Source: CAD feature listing. Evaluate the final solid. Frame: model axes, mm. A direction names the side the tool comes from. Give positions to 0.01 mm unless a question says otherwise; leave off trailing zeros. Loops run counter-clockwise (first coordinate to the right, second up) from the corner with the lowest first, then second, coordinate; pieces in that order, holes last. Notation, with made-up numbers: M -35.5,-14 L -20.5,-14 A27 ccw -20.5,16 Z; hole C -8,-7 d5. An arc over 180 degrees is marked long. Answer in a Markdown table with one row per item.
Autodesk Inventor part; units mm, degrees
ref_plane "YZ Plane" through (0, 0, 0) normal (1, 0, 0) x (0, 1, 0)
ref_plane "XZ Plane" through (0, 0, 0) normal (0, 1, 0) x (-1, 0, 0)
ref_plane "XY Plane" through (0, 0, 0) normal (0, 0, 1) x (1, 0, 0)
sketch "Sketch1" plane through (0, 0, 0) normal (0, 0, 1) x (1, 0, 0)
  line L0 (87.39809, 90.638849) -> (76.791489, 101.245451)
  line L1 (110.603697, 90.638591) -> (87.39809, 90.638849)
  line L2 (121.210063, 101.244956) -> (110.603697, 90.638591)
  line L3 (143.419374, 101.244709) -> (121.210063, 101.244956)
  line L4 (153.419263, 111.244598) -> (143.419374, 101.244709)
  line L5 (153.419473, 130.081843) -> (153.419263, 111.244598)
  line L6 (144.001258, 139.500058) -> (153.419473, 130.081843)
  line L7 (144.001258, 184.500058) -> (144.001258, 139.500058)
  line L8 (162.838724, 203.336883) -> (144.001258, 184.500058)
  line L9 (174.479779, 203.336684) -> (162.838724, 203.336883)
  line L10 (188.623093, 217.476415) -> (174.479779, 203.336684)
  line L11 (188.623904, 237.476415) -> (188.623093, 217.476415)
  line L12 (174.481567, 251.622561) -> (188.623904, 237.476415)
  line L13 (154.481567, 251.622902) -> (174.481567, 251.622561)
  line L14 (140.33919, 237.481007) -> (154.481567, 251.622902)
  line L15 (140.338992, 225.83779) -> (140.33919, 237.481007)
  line L16 (121.502223, 207.001664) -> (140.338992, 225.83779)
  line L17 (76.502223, 207.001664) -> (121.502223, 207.001664)
  line L18 (57.665842, 225.839164) -> (76.502223, 207.001664)
  line L19 (57.66604, 237.480627) -> (57.665842, 225.839164)
  line L20 (43.524145, 251.623004) -> (57.66604, 237.480627)
  line L21 (23.524145, 251.623344) -> (43.524145, 251.623004)
  line L22 (9.381769, 237.48145) -> (23.524145, 251.623344)
  line L23 (9.380958, 217.48145) -> (9.381769, 237.48145)
  line L24 (23.52252, 203.338741) -> (9.380958, 217.48145)
  line L25 (35.165328, 203.338269) -> (23.52252, 203.338741)
  line L26 (54.001421, 184.501058) -> (35.165328, 203.338269)
  line L27 (54.001421, 139.501058) -> (54.001421, 184.501058)
  line L28 (44.582671, 130.082867) -> (54.001421, 139.501058)
  line L29 (44.582461, 111.245809) -> (44.582671, 130.082867)
  line L30 (54.582226, 101.245698) -> (44.582461, 111.245809)
  line L31 (76.791489, 101.245451) -> (54.582226, 101.245698)
  circle A0 centre (99, 132) radius 5.5
  arc A1 (130.06, 142) -> (135.06, 142) centre (132.56, 142) ccw
  line L32 (130.06, 142) -> (130.06, 182)
  line L33 (135.06, 182) -> (135.06, 142)
  arc A2 (62.940969, 142) -> (67.940969, 142) centre (65.440969, 142) ccw
  arc A3 (67.940969, 182) -> (62.940969, 182) centre (65.440969, 182) ccw
  line L34 (67.940969, 182) -> (67.940969, 142)
  line L35 (138.997508, 214.221497) -> (150.997508, 202.221497)
  line L36 (128.721743, 214.221497) -> (138.997508, 214.221497)
  line L37 (121.5, 207) -> (128.721743, 214.221497)
  line L38 (76.5, 207) -> (121.5, 207)
  line L39 (69.278592, 214.221497) -> (76.5, 207)
  line L40 (59.002492, 214.221497) -> (69.278592, 214.221497)
  line L41 (47.002492, 202.221497) -> (59.002492, 214.221497)
  line L42 (47.002492, 191.497594) -> (47.002492, 202.221497)
  line L43 (54, 184.5) -> (47.002492, 191.497594)
  line L44 (54, 139.5) -> (54, 184.5)
  line L45 (47.002492, 132.502579) -> (54, 139.5)
  line L46 (47.002492, 121.778503) -> (47.002492, 132.502579)
  line L47 (59.002492, 109.778503) -> (47.002492, 121.778503)
  line L48 (69.278414, 109.778503) -> (59.002492, 109.778503)
  line L49 (76.5, 117) -> (69.278414, 109.778503)
  line L50 (121.5, 117) -> (76.5, 117)
  line L51 (128.721408, 109.778503) -> (121.5, 117)
  line L52 (138.997508, 109.778503) -> (128.721408, 109.778503)
  line L53 (150.997508, 121.778503) -> (138.997508, 109.778503)
  line L54 (150.997508, 132.502406) -> (150.997508, 121.778503)
  line L55 (144, 139.5) -> (150.997508, 132.502406)
  line L56 (144, 184.5) -> (144, 139.5)
  line L57 (150.997508, 191.497269) -> (144, 184.5)
  line L58 (150.997508, 202.221497) -> (150.997508, 191.497269)
  arc A4 (99.74629, 120.775345) -> (99.246799, 120.752769) centre (99, 131.75) ccw
  line L59 (111.585786, 133.75) -> (111, 133.75)
  line L60 (111.585786, 133.75) -> (111.585786, 135.25)
  line L61 (111.585786, 135.25) -> (113.5, 135.25)
  line L62 (113.5, 135.45) -> (113.5, 135.25)
  line L63 (113.5, 135.45) -> (113.917157, 135.45)
  line L64 (113.917157, 135.45) -> (113.917157, 141.55)
  line L65 (110.05, 169.167157) -> (103.95, 169.167157)
  line L66 (103.95, 169.167157) -> (103.95, 166.667157)
  line L67 (103.95, 166.667157) -> (94.05, 166.667157)
  line L68 (94.05, 166.667157) -> (94.05, 169.167157)
  line L69 (87.95, 169.167157) -> (87.95, 168.75)
  line L70 (87.95, 168.75) -> (87.5, 168.75)
  line L71 (86.414214, 135.25) -> (84.5, 135.25)
  line L72 (86.414214, 135.25) -> (86.414214, 133.75)
  line L73 (86.414214, 133.75) -> (87, 133.75)
  line L74 (87, 133.75) -> (87, 125.5)
  line L75 (87, 125.5) -> (89, 125.5)
  line L76 (109, 125.5) -> (111, 125.5)
  line L77 (111, 125.5) -> (111, 133.75)
  line L78 (85, 136.25) -> (86, 136.25)
  line L79 (86, 136.25) -> (86, 137.354356)
  line L80 (104.686492, 167.25) -> (104.686492, 168.25)
  line L81 (104.686492, 168.25) -> (105.854356, 168.25)
  line L82 (105.854356, 167.25) -> (104.686492, 167.25)
  circle A5 centre (99, 131.75) radius 11
  point P0 (0, 0)
  point P1 (0, 0)
extrude "Extrusion1" add sketch "Sketch1" along normal blind 5 contours L0 L31 L30 L29 L28 L46 L47 L48 L49 L50 L51 L52 L53 L54 L6 L5 L4 L3 L2 L1 | L28 L27 L26 L42 L41 L40 L39 L17 L16 L36 L35 L58 L8 L7 L6 L54 L53 L52 L51 L50 L49 L48 L47 L46 | L26 L25 L24 L23 L22 L21 L20 L19 L18 L39 L40 L41 L42 | L58 L35 L36 L16 L15 L14 L13 L12 L11 L10 L9 L8 | A0 | A5 A4
extrude "Extrusion2" add sketch "Sketch1" along normal blind 50.4 contours L28 L27 L26 L42 L41 L40 L39 L17 L16 L36 L35 L58 L8 L7 L6 L54 L53 L52 L51 L50 L49 L48 L47 L46 | A0 | A5 A4
extrude "Extrusion3" add sketch "Sketch1" along normal blind 87.4 contours A0 | A5 A4
sketch "Sketch2" plane through (0, 0, 50.4) normal (0, 0, 1) x (1, 0, 0)
  circle A0 centre (99, 131.75) radius 11
  line L0 (144, 184.5) -> (144, 139.5)
  line L1 (99, 120.75) -> (112, 120.75)
  line L2 (112, 120.75) -> (112, 165.75)
  line L3 (112, 165.75) -> (86, 165.75)
  line L4 (86, 165.75) -> (86, 120.75)
  line L5 (86, 120.75) -> (99, 120.75)
  point P0 (0, 0)
  dimension "d6" = 13
  dimension "d7" = 45
  dimension "d8" = 26
extrude "Extrusion4" add sketch "Sketch2" along normal blind 34
fillet "Fillet1" radius 2 7 edges at (112, 165.75, 67.4) (112, 143.25, 84.4) (112, 120.75, 67.4) (86, 120.75, 67.4) (86, 143.25, 84.4) (99, 165.75, 84.4) (86, 165.75, 67.4)
sketch "Sketch3" plane through (150.997508, 191.497269, 5) normal (1, 0, 0) x (0, 0, -1)
  line L0 (0, 10.724228) -> (0, 0)
  line L1 (0, 0) -> (-45.4, 0)
  line L2 (0, 10.724228) -> (0, 62.129515)
  line L3 (0, 62.129515) -> (15.429551, 62.129515)
  line L4 (15.429551, 62.129515) -> (15.429551, -102.504069)
  line L5 (15.429551, -102.504069) -> (0, -102.504069)
  line L6 (0, -102.504069) -> (0, 10.724228)
  point P0 (5, -191.497269)
extrude "Extrusion5" cut sketch "Sketch3" along normal through all both and the other way through all
properties part number "Base_NOBOTTOMPLATE"
Q1. Ray query, probe 1 along Y at (x, z) = (87.5, 50); probe 2 along Y at (x, z) = (98, 54.5); probe 3 along X at (y, z) = (139, 77.5). Return the intervals inside material, ascending. Write a range as from..to.
Values follow:
| item | result |
|---|---|
| probe 1 | 117..207 |
| probe 2 | 120.75..165.75 |
| probe 3 | 86..112 |
Q2. Section query C-C (x = 94.5). Output: boundary loops of the cut face in (y, z).
Values follow:
| item | result |
|---|---|
| outline | M 117,5 L 207,5 L 207,50.4 L 165.75,50.4 L 165.75,82.4 A2 ccw 163.75,84.4 L 141.79,84.4 L 141.79,87.4 L 121.71,87.4 L 121.71,84.4 L 120.75,84.4 L 120.75,50.4 L 117,50.4 Z |
Q3. Reachability of faces 1 (the flat face through (147.45, 136.05, 27.38)), 2 (the flat face through (99, 165.75, 66)), 3 (the flat face through (72.8, 210.7, 27.4)), 4 (the flat face through (99, 120.75, 67)), 5 (the flat face through (72.9, 113.4, 27.4)) from +Z, -Z, +X, -X, +Y, -Y: full face, straight path, thin tool, end or side. Return the list, or none.
Values follow:
| item | result |
|---|---|
| face 1 | +Z, -Z, +X |
| face 2 | +Z, +X, -X, +Y |
| face 3 | +Z, -Z, +Y |
| face 4 | +Z, +X, -X, -Y |
| face 5 | +Z, -Z, -Y |
Q4. Mould query, pull axis Y, two halves, no side actions, for faces 6 (the flat face through (150.998, 197, 27)), 7 (the flat face through (64, 109.779, 27)), 8 (the flat face through (50.5, 136, 27.4)). Classes: +Y half, -Y half, draft (parallel to the pull), parting line (faces both ways), or undercut.
Values follow:
| item | result |
|---|---|
| face 6 | draft |
| face 7 | -Y half |
| face 8 | undercut |
Q5. Section query B-B (y = 176). Output: boundary loops of the cut face in (x, z), plus the area to 3 significant figures.
Values follow:
| item | result |
|---|---|
| outline | M 54,5 L 144,5 L 144,50.4 L 54,50.4 Z |
| area | 4,090 mm^2 |
Q6. Section query A-A (z = 65.5). Output: boundary loops of the cut face in (x, y), plus the area to 3 significant figures.
Values follow:
| item | result |
|---|---|
| outline | M 86,122.75 A2 ccw 88,120.75 L 110,120.75 A2 ccw 112,122.75 L 112,163.75 A2 ccw 110,165.75 L 88,165.75 A2 ccw 86,163.75 Z |
| area | 1,170 mm^2 |
Q7. Contact query for flat-ended pins moving along their axis: pin 1 Ø4 at (y, z) = (168, 49) entering from -X; pin 2 Ø9.5 at (y, z) = (142, 72.5) entering from +X; pin 3 Ø17.5 at (x, y) = (101, 153) entering from +Z. Output: stop coordinate, or through.
Values follow:
| item | result |
|---|---|
| pin 1 | x = 54 |
| pin 2 | x = 112 |
| pin 3 | z = 84.4 |
Q8. Section query D-D (z = 23). Output: boundary loops of the cut face in (x, y), plus the area to 3 significant figures.
Values follow:
| item | result |
|---|---|
| outline | M 47,121.78 L 59,109.78 L 69.28,109.78 L 76.5,117 L 121.5,117 L 128.72,109.78 L 139,109.78 L 151,121.78 L 151,132.5 L 144,139.5 L 144,184.5 L 151,191.5 L 151,202.22 L 139,214.22 L 128.72,214.22 L 121.5,207 L 76.5,207 L 69.28,214.22 L 59,214.22 L 47,202.22 L 47,191.5 L 54,184.5 L 54,139.5 L 47,132.5 Z |
| area | 9,090 mm^2 |
